Geometry: see drawing. Coordinates: mm, zero at the bounding-box minimum. Give positions to 0.01 mm unless a question says otherwise; leave off trailing zeros. Write each loop counter-clockwise with the first axis right and the second up, starting at its lowest first coordinate (ties: lowest second). Pieces come first, ordered by that corner, then holes. Notation, with made-up numbers: (1, -20) -> (32, -20) arc R12 cw to (32, -9) -> close; hole circle Ø9 at (35.25, 86.5). An arc over 180 degrees is marked (long way). Answer as a JSON object with one key per item and string values. Group by question number.
Item 1: Ray query, probe 1 along X at (y, z) = (6.35, 2.3); probe 2 along Y at (x, z) = (12.7, 1.65); probe 3 along X at (y, z) = (33, 0.95). Return the intervals inside material, ascending. Write a range as from..to.
Item 2: First-contact query: pin 1 Ø5.5 at (x, y) = (115.47, 31.75) entering from +Z. Flat tip, straight axial feed; report the tip coordinate or a pass-through.
Item 3: Section query C-C on x = 12.7. Return the cut outline in (y, z) (1 decimal).
Item 4: Section query B-B on y = 6.35. Return the cut outline in (x, z) (1 decimal).
Item 5: Section query A-A on z = 2.15. Give the number of separate pieces and of enclosed holes in the cut face, plus the area to 3 significant figures.
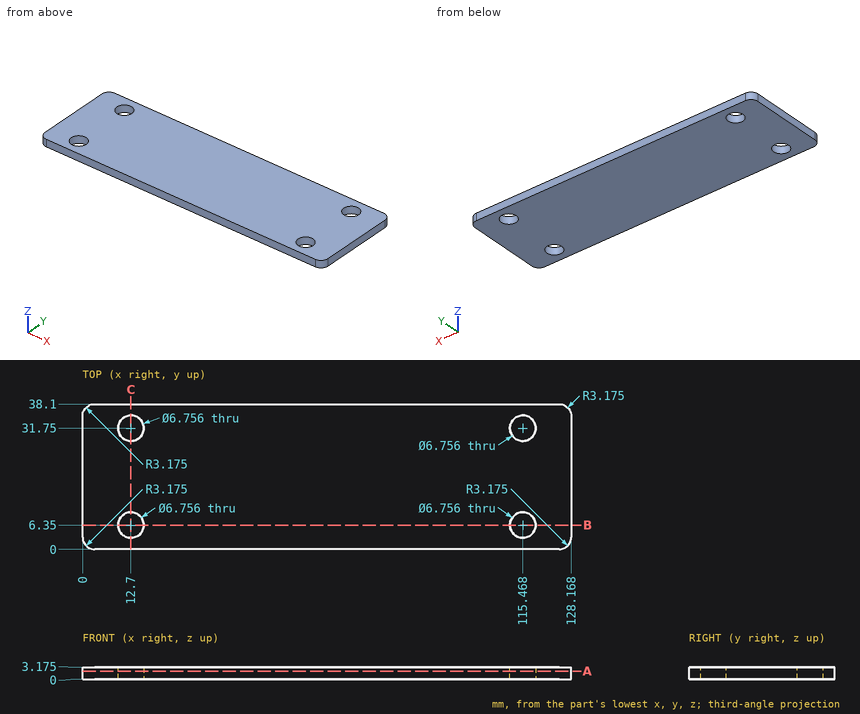
Worked answers:
{
 "1": {"probe 1": "0..9.32, 16.08..112.09, 118.85..128.17", "probe 2": "0..2.97, 9.73..28.37, 35.13..38.1", "probe 3": "0..9.56, 15.84..112.33, 118.61..128.17"},
 "2": {"pin 1": "through"},
 "3": {"outline": "(0, 0) -> (3, 0) -> (3, 3.2) -> (0, 3.2) -> close; (9.7, 0) -> (28.4, 0) -> (28.4, 3.2) -> (9.7, 3.2) -> close; (35.1, 0) -> (38.1, 0) -> (38.1, 3.2) -> (35.1, 3.2) -> close"},
 "4": {"outline": "(0, 0) -> (9.3, 0) -> (9.3, 3.2) -> (0, 3.2) -> close; (16.1, 0) -> (112.1, 0) -> (112.1, 3.2) -> (16.1, 3.2) -> close; (118.8, 0) -> (128.2, 0) -> (128.2, 3.2) -> (118.8, 3.2) -> close"},
 "5": {"separate pieces": "1", "enclosed holes": "4", "area": "4,730 mm^2"}
}
